Verification items for the finished model (mm, model axes). A direction names the side the tool comes from. Round coordinates to 2 decimals unless told otherwise and drop trailing zeros. Write each loop counter-clockwise with the first axis right and the second up, starting at its lowest first coordinate (ties: lowest second). Pieces come first, ordered by that corner, then holes. Notation, with made-up numbers: M 77,48 L 132,48 A30 cw 132,86 Z; hole C 62.5,82 d11. An arc over 180 degrees is marked long. One line per item, written item: value. Start each with the question number.
from build123d import *

# Parameters (mm, degrees)
SKETCH1_R           = 33
BOSS_EXTRUDE1_DEPTH = 3
BOSS_EXTRUDE2_DEPTH = 28
CIRPATTERN1_COUNT   = 4
SKETCH5_R           = 4.75
BOSS_EXTRUDE3_DEPTH = 40


with BuildPart() as part:
    # Sketch1 → Boss-Extrude1 (new body)
    with BuildSketch(Plane(origin=(0, 0, 0), x_dir=(1, 0, 0), z_dir=(0, 1, 0))):
        with Locations(Location((0, 0, 0), (0, 0, 270))):
            Circle(SKETCH1_R)
    extrude(amount=BOSS_EXTRUDE1_DEPTH)

    # Sketch2 → Boss-Extrude2 (add)
    with BuildSketch(Plane(origin=(0, 3, 0), x_dir=(1, 0, 0), z_dir=(0, 1, 0))):
        with BuildLine():
            ThreePointArc((1.5, 32.965891464), (0.750193874, 32.991471764), (0, 33))
            Line((0, 33), (0, 8))
            Line((0, 8), (1.5, 8))
            Line((1.5, 8), (1.5, 32.965891464))
        make_face()
        with BuildLine():
            Line((0, 8), (0, 33))
            ThreePointArc((0, 33), (-0.750193874, 32.991471764), (-1.5, 32.965891464))
            Line((-1.5, 32.965891464), (-1.5, 8))
            Line((-1.5, 8), (0, 8))
        make_face()
    boss_extrude2 = extrude(amount=BOSS_EXTRUDE2_DEPTH)

    # CirPattern1: Boss-Extrude2 ×4 about axis
    cirpattern1_axis = Axis((0, 0, 0), (0, 1, 0))
    for i in range(1, CIRPATTERN1_COUNT):
        add(boss_extrude2.rotate(cirpattern1_axis, i * 360 / CIRPATTERN1_COUNT))

    # Sketch5 → Boss-Extrude3 (add)
    with BuildSketch(Plane.XZ):
        with Locations(Location((0, 0, 0), (0, 0, 90))):
            Circle(SKETCH5_R)
    extrude(amount=BOSS_EXTRUDE3_DEPTH)

    # Sketch6 → Cut-Revolve1 (revolve, cut)
    with BuildSketch(Plane.XY, mode=Mode.PRIVATE) as cut_revolve1_sk:
        Polygon((-4.75, -16), (-3.75, -17), (-3.75, -21), (-4.75, -22), align=None)
    revolve(cut_revolve1_sk.sketch.rotate(Axis((0, 0, 0), (0, -1, 0)), 270), axis=Axis((0, 0, 0), (0, -1, 0)), mode=Mode.SUBTRACT)


solid = part.part
1) Cross-section at B-B (x = 18.5). Record the boundary of the cut face in (y, z).
2) Gauge pin test, flat ends, axial feed: pin 1 Ø5 at (x, y) = (-9.5, 15) entering from -Z; pin 2 Ø20 at (y, z) = (23.5, -24.5) entering from +X; pin 3 Ø5 at (x, z) = (-15.5, 24) entering from -Y; pin 4 Ø0.9 at (x, y) = (-0.5, 23.5) entering from -Z. Record the tip position at first contact, or that the pin passes through.
3) Cross-section at A-A (y = 4). Record the boundary of the cut face in (x, z).
4) Thickness scan on line 1 (Y direction, x = 18, z = -1); line 2 (X direction, y = 22, z = -1); line 3 (Y direction, x = -29, z = -3). Record the ranges inside material, lowest first.
5) Access from +Z, -Z, +X, -X, +Y, -Y to the whole of each face (thin tool, end or side, straight path). Record for faces 5 (the flat face through (1.5, 17, -20)), 6 (the flat face through (0, 17, 8)), 7 (the flat face through (-20, 17, -1.5)), 8 (the flat face through (-21, 17, 1.5)), 9 (the flat face through (-1.5, 17, -21)).
6) Mould release check, pull along X, two halves, no side actions. Record for faces 1 (the flat face through (-8, 17, 0)), 2 (the cylindrical face through (2.89, -30.87, -3.77)), 3 (the flat face through (-1.5, 17, 20)), 4 (the flat face through (8, 17, 0)): pulls with the +X half, pulls with the -X half, needs draft (parallel to the pull), parting line crosses it, or undercut.
7) Cross-section at C-C (z = -21). Record the boundary of the cut face in (x, y), then the cut area to 3 significant figures.
8) Cross-section at D-D (y = -25.5). Record the boundary of the cut face in (x, z), then the cut area to 3 significant figures.
Results below:
1. outline: M 0,-27.33 L 3,-27.33 L 3,-1.5 L 31,-1.5 L 31,1.5 L 3,1.5 L 3,27.33 L 0,27.33 Z
2. pin 1: stops at z = -1.5
2. pin 2: stops at x = 1.5
2. pin 3: stops at y = 0
2. pin 4: stops at z = -33
3. outline: M -32.97,-1.5 L -8,-1.5 L -8,1.5 L -32.97,1.5 A33 ccw Z; M -1.5,-32.97 A33 ccw 1.5,-32.97 L 1.5,-8 L -1.5,-8 Z; M -1.5,8 L 1.5,8 L 1.5,32.97 A33 ccw -1.5,32.97 Z; M 8,-1.5 L 32.97,-1.5 A33 ccw 32.97,1.5 L 8,1.5 Z
4. line 1: y = 0 to 31
4. line 2: x = -32.98 to -8, 8 to 32.98
4. line 3: y = 0 to 3
5. face 5: +Z, -Z, +X, +Y
5. face 6: +X, -X, +Y
5. face 7: -Z, +X, -X, +Y
5. face 8: +Z, +X, -X, +Y
5. face 9: +Z, -Z, -X, +Y
6. face 1: undercut
6. face 2: parting line crosses it
6. face 3: pulls with the -X half
6. face 4: undercut
7. outline: M -25.46,0 L 25.46,0 L 25.46,3 L 1.5,3 L 1.5,31 L -1.5,31 L -1.5,3 L -25.46,3 Z
7. area: 237 mm²
8. outline: C 0,0 d9.5
8. area: 70.9 mm²
